from build123d import *

# Parameters (mm, degrees)
F4_D = 25.4


# Not quite as in the source:
# - a fillet or chamfer that OpenCascade refuses, or shapes differently, is made with other operations: its cross-section is extruded or revolved along the edge and cut away or added


with BuildPart() as f1:
    # F0 (on Front) → F1 (revolve)
    with BuildSketch(Plane.XZ):
        Polygon((-33.655, 107.95), (-40.005, 107.95), (-48.8566160202, 107.95), (-48.8566160202, 104.1120141745), (-40.005, 91.8462350965), (-40.005, 0), (0, 0), (0, 6.35), (-33.655, 6.35), align=None)
    revolve(axis=Axis((0, 0, 3.175), (0, 0, -1)))

    # F2: fillet of radius 5.08 on 2 edges, made by hand

    # F2_s1 → F2_t2 (revolve, cut)
    with BuildSketch(Plane.XZ):
        with BuildLine():
            ThreePointArc((-33.655, 102.87), (-35.1428975516, 106.4621024484), (-38.735, 107.95))
            Line((-38.735, 107.95), (-33.655, 107.95))
            Line((-33.655, 107.95), (-33.655, 102.87))
        make_face()
    revolve(axis=Axis((0, 0, 107.95), (0, 0, -1)), mode=Mode.SUBTRACT)

    # F2_s3 → F2_t4 (revolve, cut)
    with BuildSketch(Plane.XZ):
        with BuildLine():
            ThreePointArc((-43.9307860606, 107.95), (-47.0530422956, 106.8772329609), (-48.8566160202, 104.1120141745))
            Line((-48.8566160202, 104.1120141745), (-48.8566160202, 107.95))
            Line((-48.8566160202, 107.95), (-43.9307860606, 107.95))
        make_face()
    revolve(axis=Axis((0, 0, 107.95), (0, 0, -1)), mode=Mode.SUBTRACT)

    # F4 (through all)
    with Locations(Plane(origin=(0, 0, 0), x_dir=(1, 0, 0), z_dir=(0, 0, -1))):
        with Locations((0, 0)):
            Hole(F4_D / 2)


solid = f1.part
Source: CAD feature listing. Evaluate the final solid. Frame: model axes, mm. A direction names the side the tool comes from. Coordinates: 2 decimals unless noted, no trailing zeros. Order: outer loops, then holes, each group sorted by start corner. A loop starts at its lowest first (then second) coordinate and runs counter-clockwise, first axis right, second up. Notation, with made-up numbers: M 5.5,-10 L 42.5,-10 A19 cw 42.5,9 Z; hole C 36,56 d9. An arc over 180 degrees is marked long. Write each question's results on one line, items separated by ' | '. Start each with the question number.
Item 1: Cut plane A-A (y = 0). Return loops of the section in (x, z) (3 decimals), and give its area (3 significant figures).
Item 2: Cut plane C-C (z = 84). Return loops of the section in (x, y) (3 decimals).
Item 3: Line query: probe 1 along Y at (x, z) = (0, 1.5) (3 decimals); probe 2 along Y at (x, z) = (0, 69.5) (3 decimals); probe 3 along X at (y, z) = (0.5, 37). Output: solid intervals per line, ascending.
Item 4: Draft query along Y for faces 1 (the face through (7.296, -32.855, 55.286)), 2 (the face through (0, -39, 107.95)), 3 (the face through (-38.158, 12.016, 45.28)). Return one class per face: pulls with the +Y half, pulls with the -Y half, needs draft (parallel to the pull), parting line crosses it, or undercut.
Item 5: First-contact query: pin 1 Ø12 at (y, z) = (-1.5, 22.5) entering from +X (3 decimals); pin 2 Ø2 at (x, y) = (-38.5, -30) entering from -Z; pin 3 Ø1 at (x, y) = (29, -37) entering from +Z; pin 4 Ø20.5 at (x, y) = (0, 0) entering from +Z. Flat tips, straight axial feed; report the tip coordinate or a pass-through.
Item 6: Set-up query: faces 4 (the face through (9.5, 9.5, 0)), 5 (the face through (14, 0, 6.35)). Return all of +Z, -Z, +X, -X, +Y, -Y with unobstructed straight access to the full face (end or side cutting, diameter ignored); none if empty.
Checked values:
1) outline: M -48.857,104.112 L -40.005,91.846 L -40.005,0 L -12.7,0 L -12.7,6.35 L -33.655,6.35 L -33.655,102.87 A5.08 ccw -38.735,107.95 L -43.931,107.95 A5.08 ccw Z; M 12.7,0 L 40.005,0 L 40.005,91.846 L 48.857,104.112 A5.08 ccw 43.931,107.95 L 38.735,107.95 A5.08 ccw 33.655,102.87 L 33.655,6.35 L 12.7,6.35 Z | area: 1,790 mm2
2) outline: C 0,0 d80.01; hole C 0,0 d67.31
3) probe 1: y = -40.005 to -12.7, 12.7 to 40.005 | probe 2: y = -40.005 to -33.655, 33.655 to 40.005 | probe 3: x = -40 to -33.65, 33.65 to 40
4) face 1: undercut | face 2: needs draft | face 3: parting line crosses it
5) pin 1: stops at x = 40.005 | pin 2: stops at z = 102.66 | pin 3: stops at z = 107.25 | pin 4: passes through
6) face 4: -Z, +X, -X, +Y, -Y | face 5: +Z
